from build123d import *

# Parameters (mm, degrees)
F1_DEPTH = 12
F2_DEPTH = 25
F3_DEPTH = 5
F4_R     = 4.99999


# Not quite as in the source:
# - a fillet or chamfer is up to 0.001 mm smaller than in the source, because OpenCascade refuses the exact size


with BuildPart() as f1:
    # F0 (on Top) → F1 (new body)
    with BuildSketch(Plane.XY):
        with BuildLine():
            Line((-45.8308390021, -20.6945241443), (-45.8308390021, -51.6945241443))
            Line((-45.8308390021, -51.6945241443), (42.9120542584, 56.586124615))
            Line((42.9120542584, 56.586124615), (42.9120542584, 60.586124615))
            Line((42.9120542584, 60.586124615), (33.7120542584, 60.586124615))
            Line((33.7120542584, 60.586124615), (33.7120542584, 58.1829414275))
            ThreePointArc((33.7120542584, 58.1829414275), (30.2088163179, 52.736124615), (26.7055783775, 58.1829414275))
            Line((26.7055783775, 58.1829414275), (26.7055783775, 60.586124615))
            Line((26.7055783775, 60.586124615), (17.5055783775, 60.586124615))
            Line((17.5055783775, 60.586124615), (17.5055783775, 56.586124615))
            Line((17.5055783775, 56.586124615), (-45.8308390021, -20.6945241443))
        make_face()
        with BuildLine():
            ThreePointArc((-27.6003750582, -21.0494093167), (-33.898601194, -21.7061227773), (-34.6189265027, -15.4148545048))
            Line((-34.6189265027, -15.4148545048), (-21.9413703226, 0.0538096037))
            ThreePointArc((-21.9413703226, 0.0538096037), (-15.5862024886, 0.7814511592), (-14.9228188782, -5.5807452082))
            Line((-14.9228188782, -5.5807452082), (-27.6003750582, -21.0494093167))
        make_face(mode=Mode.SUBTRACT)
        with BuildLine():
            ThreePointArc((-6.9814485555, 4.0654451881), (-13.2796746913, 3.4087317275), (-14, 9.7))
            Line((-14, 9.7), (-1.3224438199, 25.1686641085))
            ThreePointArc((-1.3224438199, 25.1686641085), (5.0327240141, 25.896305664), (5.6961076246, 19.5341092966))
            Line((5.6961076246, 19.5341092966), (-6.9814485555, 4.0654451881))
        make_face(mode=Mode.SUBTRACT)
        with BuildLine():
            ThreePointArc((13.6374779472, 29.1802996929), (7.3392518114, 28.5235862323), (6.6189265027, 34.8148545048))
            Line((6.6189265027, 34.8148545048), (19.2964826828, 50.2835186133))
            ThreePointArc((19.2964826828, 50.2835186133), (25.6516505168, 51.0111601688), (26.3150341273, 44.6489638014))
            Line((26.3150341273, 44.6489638014), (13.6374779472, 29.1802996929))
        make_face(mode=Mode.SUBTRACT)
        Polygon((-54.4308390021, -51.6945241443), (-54.4308390021, -23.6945241443), (-47.8308390021, -23.6945241443), (-47.8308390021, -51.6945241443), (-45.8308390021, -51.6945241443), (-45.8308390021, -20.6945241443), (-56.4308390021, -20.6945241443), (-56.4308390021, -51.6945241443), align=None)
    extrude(amount=F1_DEPTH)

    # F0 (on Top) → F2 (cut)
    with BuildSketch(Plane.XY):
        with BuildLine():
            Line((-21.9413703226, 0.0538096037), (-34.6189265027, -15.4148545048))
            ThreePointArc((-34.6189265027, -15.4148545048), (-33.898601194, -21.7061227773), (-27.6003750582, -21.0494093167))
            Line((-27.6003750582, -21.0494093167), (-14.9228188782, -5.5807452082))
            ThreePointArc((-14.9228188782, -5.5807452082), (-15.5862024886, 0.7814511592), (-21.9413703226, 0.0538096037))
        make_face()
        with BuildLine():
            Line((-1.3224438199, 25.1686641085), (-14, 9.7))
            ThreePointArc((-14, 9.7), (-13.2796746913, 3.4087317275), (-6.9814485555, 4.0654451881))
            Line((-6.9814485555, 4.0654451881), (5.6961076246, 19.5341092966))
            ThreePointArc((5.6961076246, 19.5341092966), (5.0327240141, 25.896305664), (-1.3224438199, 25.1686641085))
        make_face()
        with BuildLine():
            Line((19.2964826828, 50.2835186133), (6.6189265027, 34.8148545048))
            ThreePointArc((6.6189265027, 34.8148545048), (7.3392518114, 28.5235862323), (13.6374779472, 29.1802996929))
            Line((13.6374779472, 29.1802996929), (26.3150341273, 44.6489638014))
            ThreePointArc((26.3150341273, 44.6489638014), (25.6516505168, 51.0111601688), (19.2964826828, 50.2835186133))
        make_face()
    extrude(amount=-F2_DEPTH, mode=Mode.SUBTRACT)

    # F0 (on Top) → F3 (cut)
    with BuildSketch(Plane.XY):
        with BuildLine():
            Line((-45.8308390021, -20.6945241443), (-45.8308390021, -51.6945241443))
            Line((-45.8308390021, -51.6945241443), (42.9120542584, 56.586124615))
            Line((42.9120542584, 56.586124615), (42.9120542584, 60.586124615))
            Line((42.9120542584, 60.586124615), (33.7120542584, 60.586124615))
            Line((33.7120542584, 60.586124615), (33.7120542584, 58.1829414275))
            ThreePointArc((33.7120542584, 58.1829414275), (30.2088163179, 52.736124615), (26.7055783775, 58.1829414275))
            Line((26.7055783775, 58.1829414275), (26.7055783775, 60.586124615))
            Line((26.7055783775, 60.586124615), (17.5055783775, 60.586124615))
            Line((17.5055783775, 60.586124615), (17.5055783775, 56.586124615))
            Line((17.5055783775, 56.586124615), (-45.8308390021, -20.6945241443))
        make_face()
        with BuildLine():
            ThreePointArc((-27.6003750582, -21.0494093167), (-33.898601194, -21.7061227773), (-34.6189265027, -15.4148545048))
            Line((-34.6189265027, -15.4148545048), (-21.9413703226, 0.0538096037))
            ThreePointArc((-21.9413703226, 0.0538096037), (-15.5862024886, 0.7814511592), (-14.9228188782, -5.5807452082))
            Line((-14.9228188782, -5.5807452082), (-27.6003750582, -21.0494093167))
        make_face(mode=Mode.SUBTRACT)
        with BuildLine():
            ThreePointArc((-6.9814485555, 4.0654451881), (-13.2796746913, 3.4087317275), (-14, 9.7))
            Line((-14, 9.7), (-1.3224438199, 25.1686641085))
            ThreePointArc((-1.3224438199, 25.1686641085), (5.0327240141, 25.896305664), (5.6961076246, 19.5341092966))
            Line((5.6961076246, 19.5341092966), (-6.9814485555, 4.0654451881))
        make_face(mode=Mode.SUBTRACT)
        with BuildLine():
            ThreePointArc((13.6374779472, 29.1802996929), (7.3392518114, 28.5235862323), (6.6189265027, 34.8148545048))
            Line((6.6189265027, 34.8148545048), (19.2964826828, 50.2835186133))
            ThreePointArc((19.2964826828, 50.2835186133), (25.6516505168, 51.0111601688), (26.3150341273, 44.6489638014))
            Line((26.3150341273, 44.6489638014), (13.6374779472, 29.1802996929))
        make_face(mode=Mode.SUBTRACT)
    extrude(amount=F3_DEPTH, mode=Mode.SUBTRACT)

    # F4 (radius 5 in the source; OpenCascade refuses exactly that, so slightly less here)
    f4_edges = [f1.edges().sort_by_distance(p)[0] for p in [
        (-45.830839, -36.194524, 5),
    ]]
    fillet(f4_edges, radius=F4_R)


solid = f1.part
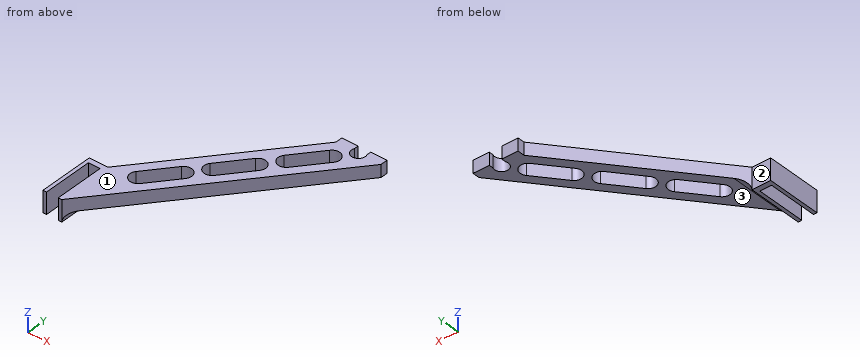
Work out the finished part from the listing and answer in its coordinate system (mm). Face numbers are marked on the shaded views. A direction names the side the tool comes from. Coordinates: 2 decimals unless noted, no trailing zeros. Order: outer loops, then holes, each group sorted by start corner. A loop starts at its lowest first (then second) coordinate and runs counter-clockwise, first axis right, second up. Notation, with made-up numbers: (21.25, -33.5) - (41.25, -33.5) arc R15 cw to (41.25, -23.5) - close; hole circle Ø5 at (-39.5, -5). An arc over 180 degrees is marked (long way). Put each result on its own line as item: value. Start each with the question number.
1) Find section B-B (y = 7.5). Give the vertices of the cut face in (x, z), plus the area to 3 significant figures.
2) For the marked faces 1, 2 and 3, determine the directions among +Z, -Z, +X, -X, +Y, -Y from which every point of the face is accessible in a straight line to the end or side of a thin tool.
3) Find the intervals of material crossed by line 1 (X direction, y = 10, z = 11.5); line 2 (X direction, y = 4, z = 10); line 3 (Y direction, x = -20, z = 10), in increasing order. Write a range as from..to.
4) Find section C-C (z = 7). Give the vertices of the cut face in (x, y), plus the area to 3 significant figures.
5) Find section A-A (x = 9). Give the vertices of the cut face in (y, z).
6) Flat-ended cylindrical pins translate along their axes: pin 1 (1 mm diameter, centred on x = -24.5, z = 10, fed in from -Y); pin 2 (2.5 mm diameter, centred on y = 59, z = 8, fed in from -X); pin 3 (6 mm diameter, centred on y = -36.5, z = 5.5, fed in from +X); pin 4 (2 mm diameter, centred on x = 1.5, z = 2.5, fed in from +Y). Find the tip coordinate at first contact, or state that the pin passes through.
Results list:
1. outline: (-22.72, 5) - (-14.92, 5) - (-14.92, 12) - (-22.72, 12) - close; (-4.17, 5) - (2.68, 5) - (2.68, 12) - (-4.17, 12) - close
1. area: 103 mm^2
2. face 1: +Z, +X, -X, +Y, -Y
2. face 2: +Z, -Z, -X, +Y
2. face 3: -Z, +X, +Y, -Y
3. line 1: x = -20.67..-13.75, -2.12..4.73
3. line 2: x = -25.59..-13.89, -7.04..-0.19
3. line 3: y = -20.18..-11.78, 1.48..10.82
4. outline: (-56.43, -51.69) - (-54.43, -51.69) - (-54.43, -23.69) - (-47.83, -23.69) - (-47.83, -51.69) - (-45.83, -51.69) - (42.91, 56.59) - (42.91, 60.59) - (33.71, 60.59) - (33.71, 58.18) arc R3.85 cw (long way) to (26.71, 58.18) - (26.71, 60.59) - (17.51, 60.59) - (17.51, 56.59) - (-45.83, -20.69) - (-56.43, -20.69) - close; hole (-34.62, -15.41) arc R4.5 ccw to (-27.6, -21.05) - (-14.92, -5.58) arc R4.5 ccw (long way) to (-21.94, 0.05) - close; hole (-14, 9.7) arc R4.5 ccw to (-6.98, 4.07) - (5.7, 19.53) arc R4.5 ccw (long way) to (-1.32, 25.17) - close; hole (6.62, 34.81) arc R4.5 ccw to (13.64, 29.18) - (26.32, 44.65) arc R4.5 ccw (long way) to (19.3, 50.28) - close
4. area: 1,820 mm^2
5. outline: (15.21, 5) - (27.68, 5) - (27.68, 12) - (15.21, 12) - close; (37.72, 5) - (46.21, 5) - (46.21, 12) - (37.72, 12) - close
6. pin 1: stops at y = -26.28
6. pin 2: stops at x = 17.51
6. pin 3: stops at x = -30.92
6. pin 4: passes through
